from build123d import *

# Parameters (mm, degrees)
F2_R     = 2.5590732694
F3_DEPTH = 10.16
F4_R     = 1.5875
F5_DEPTH = 12.7


with BuildPart() as f1:
    # F0 (on Front) → F1 (revolve)
    with BuildSketch(Plane.XZ):
        with BuildLine():
            Line((0, 36.3681837916), (0, 0))
            Line((0, 0), (1.651, 0))
            add(Edge.make_bspline(
                [(1.651, 0), (4.9784278335, 7.8432246905), (9.8797152031, 2.2916243739), (23.4813746273, 8.4736508016), (26.5273787081, 11.8374861777)],
                knots=[0, 0, 0, 0, 0.4442566338, 1, 1, 1, 1], degree=3))
            Line((26.5273787081, 11.8374861777), (26.5273787081, 26.2081837916))
            add(Edge.make_bspline(
                [(5.08, 26.2081837916), (10.0801282924, 16.6757298148), (6.5290390026, 2.9534107183), (23.0302548553, 29.295393126), (26.5273787081, 26.2081837916)],
                knots=[0, 0, 0, 0, 0.4594912223, 1, 1, 1, 1], degree=3))
            Line((5.08, 26.2081837916), (5.08, 36.3681837916))
            Line((5.08, 36.3681837916), (0, 36.3681837916))
        make_face()
    revolve(axis=Axis((0, 0, 18.1840918958), (0, 0, -1)))

    # F2 (on face) → F3 (cut)
    with BuildSketch(Plane.XY.offset(36.3681837916)):
        Circle(F2_R)
    extrude(amount=-F3_DEPTH, mode=Mode.SUBTRACT)

    # F4 (on Top) → F5 (cut)
    with BuildSketch(Plane.XY):
        Circle(F4_R)
    extrude(amount=F5_DEPTH, mode=Mode.SUBTRACT)


solid = f1.part
Verification items for the finished model (mm, model axes). A direction names the side the tool comes from. Round coordinates to 2 decimals unless told otherwise and drop trailing zeros. Order: outer loops, then holes, each group sorted by start corner. A loop starts at its lowest first (then second) coordinate and runs counter-clockwise, first axis right, second up.
1. Thickness scan on L1, parallel to Y at x = 0, z = 33; L2, parallel to X at y = 0.5, z = 13; L3, parallel to Y at x = -2.5, z = 14. Record the ranges inside material, lowest first.
Final values:
L1: y = -5.08 to -2.56, 2.56 to 5.08
L2: x = -26.52 to -11.55, -9.44 to 9.44, 11.55 to 26.52
L3: y = -26.41 to -12.23, -8.84 to 8.84, 12.23 to 26.41
2. Access from +Z, -Z, +X, -X, +Y, -Y to the whole of each face (thin tool, end or side, straight path). Record for faces 4 (the cylindrical face through (-0.34, -1.55, 6.26)), 5 (the cylindrical face through (-0.661, -5.037, 31.359)).
Final values:
face 4: -Z
face 5: +Z
3. Release check for a two-part mould opening along Y. For faces 1 (the cylindrical face through (-3.453, -26.302, 19.123)), 2 (the flat face through (2, 2, 36.368)), 3 (the flat face through (0, 0, 26.208)) record: +Y half, -Y half, draft (parallel to the pull), parting line (faces both ways), or undercut.
Final values:
face 1: parting line
face 2: draft
face 3: undercut
4. Section check A-A on z = 31. Record the cut outline in (x, y), then the cut area to 3 significant figures.
Final values:
outline: circle Ø10.16 at (0, 0); hole circle Ø5.12 at (0, 0)
area: 60.5 mm2
5. Go/stop test with flat-tipped pins: P1, Ø1, axis at x = 0, y = -0.5, coming from the -Z side; P2, Ø3, axis at x = -15, z = 21.5, coming from the -Y side; P3, Ø5, axis at x = 12.5, y = 19, coming from the +Z side. Record where each tip stops, or that it passes through.
Final values:
P1: stops at z = 12.7
P2: stops at y = -22.84
P3: stops at z = 26.64
